from build123d import *

# Parameters (mm, degrees)
BOSS_EXTRUDE1_DEPTH = 20
SKETCH2_R           = 2
CUT_EXTRUDE1_DEPTH  = 104.335618254
SKETCH4_R           = 0.5
CUT_EXTRUDE2_DEPTH  = 20


with BuildPart() as part:
    # Sketch1 → Boss-Extrude1 (new body)
    with BuildSketch(Plane.XY):
        Polygon((-24, 49.25), (0, 49.25), (0, 3.75), (20, 3.75), (20, -0.25), (0, -0.25), (0, -49.25), (-24, -49.25), (-24, -45.25), (-4, -45.25), (-4, 45.25), (-24, 45.25), align=None)
    extrude(amount=BOSS_EXTRUDE1_DEPTH)

    # Sketch2 → Cut-Extrude1 (cut, through all)
    with BuildSketch(Plane(origin=(0, 49.25, 0), x_dir=(1, 0, 0), z_dir=(0, 1, 0))):
        with Locations(Location((-18, -5, 0), (0, 0, 270))):
            Circle(SKETCH2_R)
        with Locations(Location((-10, -5, 0), (0, 0, 270))):
            Circle(SKETCH2_R)
        with Locations(Location((-10, -15, 0), (0, 0, 270))):
            Circle(SKETCH2_R)
        with Locations(Location((-18, -15, 0), (0, 0, 270))):
            Circle(SKETCH2_R)
    extrude(amount=-CUT_EXTRUDE1_DEPTH, mode=Mode.SUBTRACT)

    # Sketch4 → Cut-Extrude2 (cut)
    with BuildSketch(Plane(origin=(0, 3.75, 0), x_dir=(1, 0, 0), z_dir=(0, 1, 0))):
        with Locations(Location((15, -10, 0), (0, 0, 270))):
            Circle(SKETCH4_R)
        with Locations(Location((13, -10, 0), (0, 0, 270))):
            Circle(SKETCH4_R)
        with Locations(Location((11, -10, 0), (0, 0, 270))):
            Circle(SKETCH4_R)
        with Locations(Location((9, -10, 0), (0, 0, 270))):
            Circle(SKETCH4_R)
        with Locations(Location((7, -10, 0), (0, 0, 270))):
            Circle(SKETCH4_R)
        with Locations(Location((5, -10, 0), (0, 0, 270))):
            Circle(SKETCH4_R)
    extrude(amount=-CUT_EXTRUDE2_DEPTH, mode=Mode.SUBTRACT)


solid = part.part
Source: CAD feature listing. Evaluate the final solid. Frame: model axes, mm. A direction names the side the tool comes from. Round coordinates to 2 decimals unless told otherwise and drop trailing zeros. Loops run counter-clockwise (first coordinate to the right, second up) from the corner with the lowest first, then second, coordinate; pieces in that order, holes last. Notation, with made-up numbers: M 70,20 L 86,20 A15 cw 86,47 Z; hole C 64.25,45.25 d6. An arc over 180 degrees is marked long. Return JSON: item names as keys, results as strings. Group by question number.
1. Section query A-A on x = -18. Output: boundary loops of the cut face in (y, z).
2. Mould query, pull axis X, two halves, no side actions, for faces 4 (the face through (-16, 47, 5)), 5 (the face through (-3.5, 0.2, 0)), 6 (the face through (0, 27, 10)). Classes: released by +X, released by -X, zero draft, split by the parting line, or undercut.
3. Section query B-B on z = 12. Output: boundary loops of the cut face in (x, y), and give its area (3 significant figures).
4. Pin query (flat end, axial travel): pin 1 (1 mm diameter, centred on y = -29.5, z = 6.5, fed in from +X); pin 2 (1.5 mm diameter, centred on y = 18, z = 3, fed in from -X); pin 3 (3.5 mm diameter, centred on x = -18, z = 15, fed in from +Y). Return the tip coordinate at first contact, or that it passes through.
5. Material intervals for line 1 along X through (y, z) = (-47.1, 15); line 2 along Y through (x, z) = (-9, 1.75); line 3 along Y through (x, z) = (1.5, 14), sorted ascending. Write a range as from..to.
6. Section query C-C on y = -4.5. Output: boundary loops of the cut face in (x, z), and give its area (3 significant figures).
7. Reachability of faces 1 (the face through (-14, -45.25, 10)), 2 (the face through (10, 3.75, 10)), 3 (the face through (10, -0.25, 10)) from +Z, -Z, +X, -X, +Y, -Y: full face, straight path, thin tool, end or side. Return the list, or none.
Checks:
{
 "1": {"outline": "M -49.25,0 L -45.25,0 L -45.25,3 L -49.25,3 Z; M -49.25,7 L -45.25,7 L -45.25,13 L -49.25,13 Z; M -49.25,17 L -45.25,17 L -45.25,20 L -49.25,20 Z; M 45.25,0 L 49.25,0 L 49.25,3 L 45.25,3 Z; M 45.25,7 L 49.25,7 L 49.25,13 L 45.25,13 Z; M 45.25,17 L 49.25,17 L 49.25,20 L 45.25,20 Z"},
 "2": {"face 4": "undercut", "face 5": "zero draft", "face 6": "released by +X"},
 "3": {"outline": "M -24,-49.25 L 0,-49.25 L 0,-0.25 L 20,-0.25 L 20,3.75 L 0,3.75 L 0,49.25 L -24,49.25 L -24,45.25 L -4,45.25 L -4,-45.25 L -24,-45.25 Z", "area": "634 mm²"},
 "4": {"pin 1": "stops at x = 0", "pin 2": "stops at x = -4", "pin 3": "passes through"},
 "5": {"line 1": "x = -24..-20, -16..-12, -8..0", "line 2": "y = -49.25..-45.25, 45.25..49.25", "line 3": "y = -0.25..3.75"},
 "6": {"outline": "M -4,0 L 0,0 L 0,20 L -4,20 Z", "area": "80.0 mm²"},
 "7": {"face 1": "+Z, -Z, -X", "face 2": "+Z, -Z, +X, +Y", "face 3": "+Z, -Z, +X, -Y"}
}
